Design review of the part shown in the three views and the two pictorial views. Dimensions are in mm from the part's minimum x, y and z. A direction names the side the tool comes from. Give positions to 0.01 mm unless a question says otherwise; leave off trailing zeros. Order: outer loops, then holes, each group sorted by start corner. A loop starts at its lowest first (then second) coordinate and runs counter-clockwise, first axis right, second up. Notation, with made-up numbers: (62, -2) - (69, -2) arc R18 ccw to (69, 18) - close; hole circle Ø9 at (-39, 11). An arc over 180 degrees is marked (long way). Put each result on its own line as item: value.
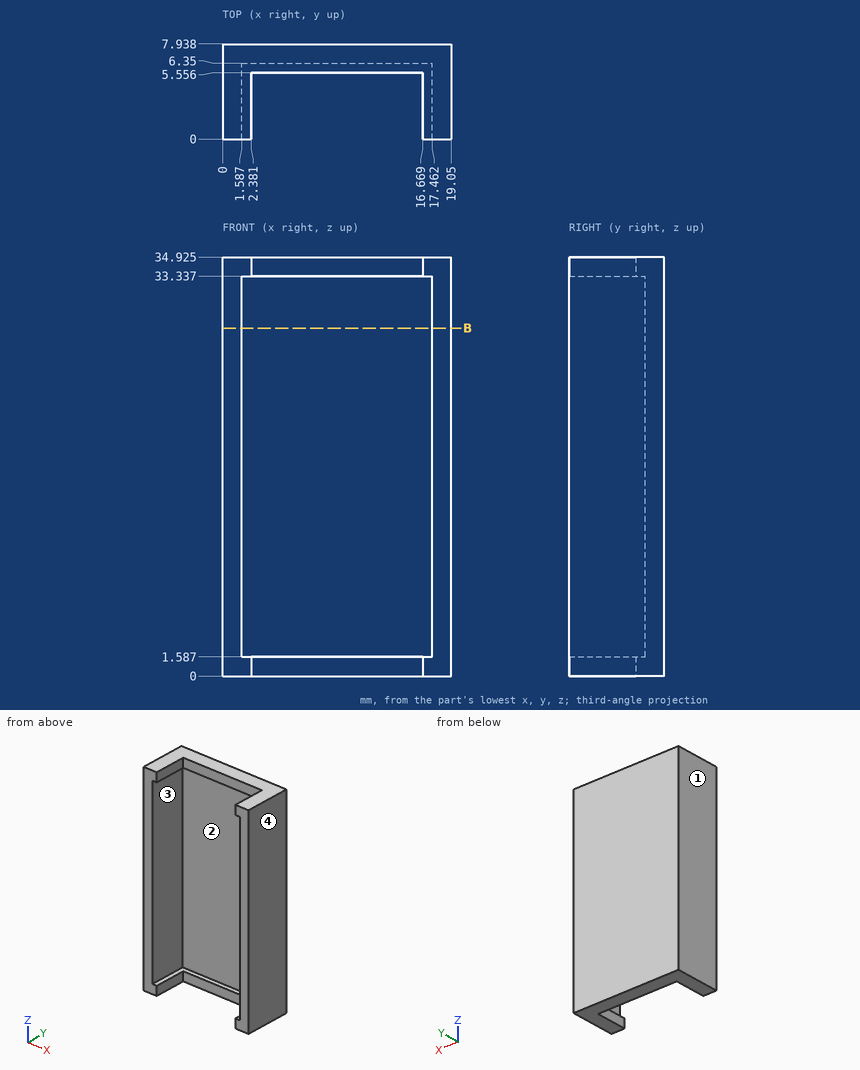
(1) The part is to be moulded in two halves that separate along Z. For the marked faces 1 and 2, say which applies: pulls with the +Z half, pulls with the -Z half, needs draft (parallel to the pull), parting line crosses it, or undercut.
The answers:
face 1: needs draft
face 2: undercut
(2) For the marked faces 3 and 4, list the 3-axis set-ups (+Z, -Z, +X, -X, +Y, -Y) from which the entire face can be reached by the end or side of a thin tool; tool diameter is ignored.
The answers:
face 3: -Y
face 4: +Z, -Z, +X, +Y, -Y
(3) Wall thickness on L1, parallel to Z at x = 7.25, y = 6.25 (1 decimal); L2, parallel to X at y = 4.25, z = 16.5; L3, parallel to Y at x = 5.5, z = 16: over which ranges is each line inside the solid? List them lowest first.
The answers:
L1: 0 to 1.6, 33.3 to 34.9
L2: 0 to 1.59, 17.46 to 19.05
L3: 6.35 to 7.94
(4) Clearance check with flat-ended pins moving along their axes: pin 1 Ø0.5 at (x, z) = (12, 34) entering from -Y; pin 2 Ø8 at (x, z) = (10, 16) entering from -Y. State where each tip first meets the part, or that it passes through.
The answers:
pin 1: y = 5.56
pin 2: y = 6.35
(5) Take a section at B-B, the plane z = 29. Write out the cut boundary in (x, y).
The answers:
outline: (0, 0) - (1.59, 0) - (1.59, 6.35) - (17.46, 6.35) - (17.46, 0) - (19.05, 0) - (19.05, 7.94) - (0, 7.94) - close
